from build123d import *

# Parameters (mm, degrees)
F1_DEPTH    = 1981.2
F2_R        = 101.6
F3_R        = 101.6
F4_T1_DEPTH = 2133.6
F4_S5_W     = 101.6
F4_S5_H     = 101.6
F4_T6_DEPTH = 101.6


# Not quite as in the source:
# - a fillet or chamfer that OpenCascade refuses, or shapes differently, is made with other operations: its cross-section is extruded or revolved along the edge and cut away or added


with BuildPart() as f1:
    # F0 (on Front) → F1 (new body)
    with BuildSketch(Plane.XZ):
        Polygon((251.7913877964, 36.7387868464), (-47.3107099533, 36.7387868464), (-47.3107099533, -855.4236292839), (777.5030732155, -855.4236292839), (777.5030732155, -434.3872666359), (251.7913877964, -434.3872666359), align=None)
    extrude(amount=F1_DEPTH)

    # F2
    f2_edges = [f1.edges().sort_by_distance(p)[0] for p in [
        (251.791388, -990.6, 36.738787),
        (-47.31071, -1981.2, -409.342421),
    ]]
    fillet(f2_edges, radius=F2_R)

    # F3
    f3_edges = [f1.edges().sort_by_distance(p)[0] for p in [
        (514.647231, -1981.2, -434.387267),
        (777.503073, -1981.2, -644.905448),
    ]]
    fillet(f3_edges, radius=F3_R)

    # F4: fillet of radius 101.6 on 1 edges, made by hand

    # F4_s2 → F4_t1 (cut)
    with BuildSketch(Plane.XZ.offset(-254)):
        with BuildLine():
            ThreePointArc((777.5030732155, -535.9872666359), (747.745122184, -464.1452176673), (675.9030732155, -434.3872666359))
            Line((675.9030732155, -434.3872666359), (777.5030732155, -434.3872666359))
            Line((777.5030732155, -434.3872666359), (777.5030732155, -535.9872666359))
        make_face()
    extrude(amount=F4_T1_DEPTH, mode=Mode.SUBTRACT)


with BuildPart() as f4_tool4:
    # F4_s5 → F4_t6 (new body)
    with BuildSketch(Plane.YZ.offset(675.9030732155)):
        with Locations((-1930.4, -485.1872666359)):
            Rectangle(F4_S5_W, F4_S5_H)
    extrude(amount=F4_T6_DEPTH)

    # F4_s7 → F4_t8 (revolve, cut)
    with BuildSketch(Plane(origin=(675.9030732155, -1879.6, -535.9872666359), x_dir=(0, 0.7071067812, -0.7071067812), z_dir=(0, -0.7071067812, -0.7071067812))):
        with BuildLine():
            ThreePointArc((0, -101.6), (101.6, 0), (0, 101.6))
            Line((0, 101.6), (0, -101.6))
        make_face()
    revolve(axis=Axis((675.9030732155, -1879.6, -535.9872666359), (1, 0, 0)), mode=Mode.SUBTRACT)


with BuildPart() as f1_1:
    add(f1.part)

    # F4_t3: cut F4_tool4
    add(f4_tool4.part, mode=Mode.SUBTRACT)


solid = f1_1.part
Geometry check sheet. Reference: the model listing, model coordinates, mm. A direction names the side the tool comes from. Round coordinates to 2 decimals unless told otherwise and drop trailing zeros. Order: outer loops, then holes, each group sorted by start corner. A loop starts at its lowest first (then second) coordinate and runs counter-clockwise, first axis right, second up. Notation, with made-up numbers: M 40,-24 L 90,-24 A36 cw 90,15 Z; hole C 71,65.5 d10. An arc over 180 degrees is marked long. Answer in a Markdown table with one row per item. Add a question column.
Item 1: Set-up check for faces 4 (the face through (777.503, -927, -698)), 5 (the face through (460.88, -1952.23, -464.94)): record each of +Z, -Z, +X, -X, +Y, -Y from which the full face is reachable in a straight line by a thin tool's end or side.
Item 2: Sectioned sample at D-D, the plane z = -456. Enter the section's corners in (x, y).
Item 3: Material ranges on L1, parallel to Z at x = 420.5, y = -243; L2, parallel to X at y = -383.5, z = -113.5; L3, parallel to Y at x = 23.5, z = -330, recorded low to high. Write a range as [from, to].
Item 4: Sectioned sample at A-A, the plane x = 629. Enter the section's corners in (y, z).
Item 5: Depth check by flat-ended pin: pin 1 Ø1.5 at (x, y) = (475, -353) entering from +Z; pin 2 Ø2 at (x, z) = (682.5, -675.5) entering from -Y. Enter the tip coordinate at first touch or a pass-through.
Item 6: Draft check along Z on faces 1 (the face through (467, -927, -434.387)), 2 (the face through (746.95, -1952.23, -693.47)), 3 (the face through (359, -977, -855.424)). Enter one of: released by +Z, released by -Z, zero draft, split by the parting line, or undercut.
Item 7: Sectioned sample at C-C, the plane z = -212. Enter the section's corners in (x, y), plus the area to 3 significant figures.
Item 8: Sectioned sample at B-B, the plane y = -909.5. Enter the section's corners in (x, z).
Filled in:
| question | item | result |
|---|---|---|
| 1 | face 4 | +Z, -Z, +X, +Y, -Y |
| 1 | face 5 | +Z, +X, -Y |
| 2 | outline | M -47.31,-1879.6 A101.6 ccw 54.29,-1981.2 L 251.79,-1981.2 L 251.79,-1942.25 L 675.9,-1942.25 A62.65 ccw 738.55,-1879.6 L 738.55,0 L -47.31,0 Z |
| 3 | L1 | z = [-855.42, -434.39] |
| 3 | L2 | x = [-47.31, 251.79] |
| 3 | L3 | y = [-1976.42, 0] |
| 4 | outline | M -1981.2,-855.42 L 0,-855.42 L 0,-434.39 L -1879.6,-434.39 A101.6 ccw -1981.2,-535.99 Z |
| 5 | pin 1 | stops at z = -434.39 |
| 5 | pin 2 | stops at y = -1981.05 |
| 6 | face 1 | released by +Z |
| 6 | face 2 | zero draft |
| 6 | face 3 | released by -Z |
| 7 | outline | M -47.31,-1879.6 A101.6 ccw 54.29,-1981.2 L 251.79,-1981.2 L 251.79,0 L -47.31,0 Z |
| 7 | area | 590,000 mm² |
| 8 | outline | M -47.31,-855.42 L 777.5,-855.42 L 777.5,-535.99 A101.6 ccw 675.9,-434.39 L 251.79,-434.39 L 251.79,-64.86 A101.6 ccw 150.19,36.74 L -47.31,36.74 Z |
